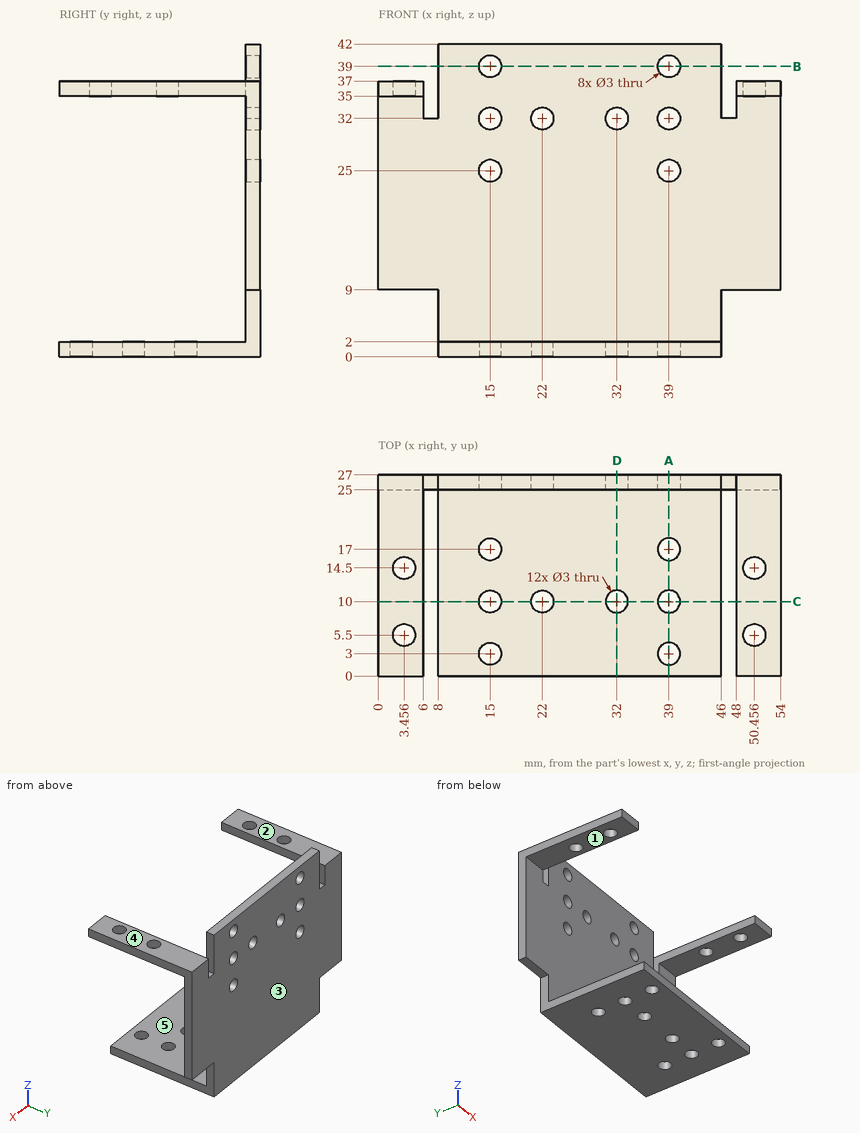
Geometry check sheet. Reference: drawing and pictorial views, mm from the part's lowest x, y, z. A direction names the side the tool comes from. Give positions to 0.01 mm unless a question says otherwise; leave off trailing zeros. Write each loop counter-clockwise with the first axis right and the second up, starting at its lowest first coordinate (ties: lowest second). Pieces come first, ordered by that corner, then holes. Notation, with made-up numbers: M 86.25,-14 L 109.25,-14 A22 ccw 109.25,18 Z; hole C 5,66.5 d9. An arc over 180 degrees is marked long. Use CSV: the item, a comma, the result in double quotes.
1) Cross-section at C-C (y = 10). Enter the section's corners in (x, z).
Final values:
outline,"M 0,35 L 6,35 L 6,37 L 0,37 Z; M 8,0 L 13.5,0 L 13.5,2 L 8,2 Z; M 16.5,0 L 20.5,0 L 20.5,2 L 16.5,2 Z; M 23.5,0 L 30.5,0 L 30.5,2 L 23.5,2 Z; M 33.5,0 L 37.5,0 L 37.5,2 L 33.5,2 Z; M 40.5,0 L 46,0 L 46,2 L 40.5,2 Z; M 48,35 L 54,35 L 54,37 L 48,37 Z"
2) Cross-section at B-B (z = 39). Enter the section's corners in (x, y).
Final values:
outline,"M 8,25 L 13.5,25 L 13.5,27 L 8,27 Z; M 16.5,25 L 37.5,25 L 37.5,27 L 16.5,27 Z; M 40.5,25 L 46,25 L 46,27 L 40.5,27 Z"
3) Access from +Z, -Z, +X, -X, +Y, -Y to the whole of each face (thin tool, end or side, straight path). Record for the marked faces 1, 2, 3, 4 and 5.
Final values:
face 1,"-Z, +X, -X, -Y"
face 2,"+Z, -X, +Y, -Y"
face 3,"+Z, -Z, +X, -X, +Y"
face 4,"+Z, +X, +Y, -Y"
face 5,"+Z, +X, -X, -Y"
4) Material ranges on line 1 along Z through (x, y) = (39, 25.6); line 2 along X through (y, z) = (25.65, 39); line 3 along X through (y, z) = (26.45, 25), recorded low to high.
Final values:
line 1,"0 to 23.5, 26.5 to 30.5, 33.5 to 37.5, 40.5 to 42"
line 2,"8 to 13.5, 16.5 to 37.5, 40.5 to 46"
line 3,"0 to 13.5, 16.5 to 37.5, 40.5 to 54"
5) Go/stop test with flat-tipped pins: pin 1 Ø3 at (x, z) = (20.5, 36.5) entering from -Y; pin 2 Ø7 at (y, z) = (12.5, 2.5) entering from +X; pin 3 Ø4 at (x, y) = (15, 3) entering from +Z. Record where each tip stops, or that it passes through.
Final values:
pin 1,"y = 25"
pin 2,"x = 46"
pin 3,"z = 2"
6) Cross-section at D-D (x = 32). Enter the section's corners in (y, z).
Final values:
outline,"M 0,0 L 8.5,0 L 8.5,2 L 0,2 Z; M 11.5,0 L 27,0 L 27,30.5 L 25,30.5 L 25,2 L 11.5,2 Z; M 25,33.5 L 27,33.5 L 27,42 L 25,42 Z"
7) Cross-section at A-A (x = 39). State how many separate pieces and enclosed holes the cut face has.
Final values:
separate pieces,"7"
enclosed holes,"0"
